Check sheet for the drawn part. Datum: minimum x, y, z corner. Units: mm. A direction names the side the tool comes from. Give positions to 0.01 mm unless a question says otherwise; leave off trailing zeros. Loops run counter-clockwise (first coordinate to the right, second up) from the corner with the lowest first, then second, coordinate; pieces in that order, holes last. Notation, with made-up numbers: (50.5, -24.75) - (86.5, -24.75) arc R21 ccw to (86.5, 2.25) - close; hole circle Ø11 at (41, -18). An arc over 180 degrees is marked (long way). One line per item, written item: value. Start each with the question number.
1. Sectioned sample at A-A (y = 3.5). Record the cut outline in (x, z), plus the area to 3 significant figures.
2. Sectioned sample at D-D (y = 0.5). Record the cut outline in (x, z).
3. Access from +Z, -Z, +X, -X, +Y, -Y to the whole of each face (thin tool, end or side, straight path). Record for the marked faces 1, 2 and 3.
4. Gauge pin test, flat ends, axial feed: pin 1 (1.6 mm diameter, centred on y = 4.5, z = 9, fed in from +X); pin 2 (2 mm diameter, centred on x = 7.5, y = 2.5, fed in from +Z). Record the tip position at first contact, or that the pin passes through.
5. Scan lines: L1, parallel to Z at x = 1, y = 3.5; L2, parallel to X at y = 2.5, z = 5.5; L3, parallel to Y at x = 0.5, z = 9. Record each from-to range of solid material in increasing order. Write a range as [from, to].
6. Mould release check, pull along X, two halves, no side actions. Record for the marked faces 4, 5, 6 and 7: pulls with the +X half, pulls with the -X half, needs draft (parallel to the pull), parting line crosses it, or undercut.
7. Sectioned sample at C-C (z = 10). Record the cut outline in (x, y), plus the area to 3 significant figures.
8. Sectioned sample at B-B (z = 12). Record the cut outline in (x, y).
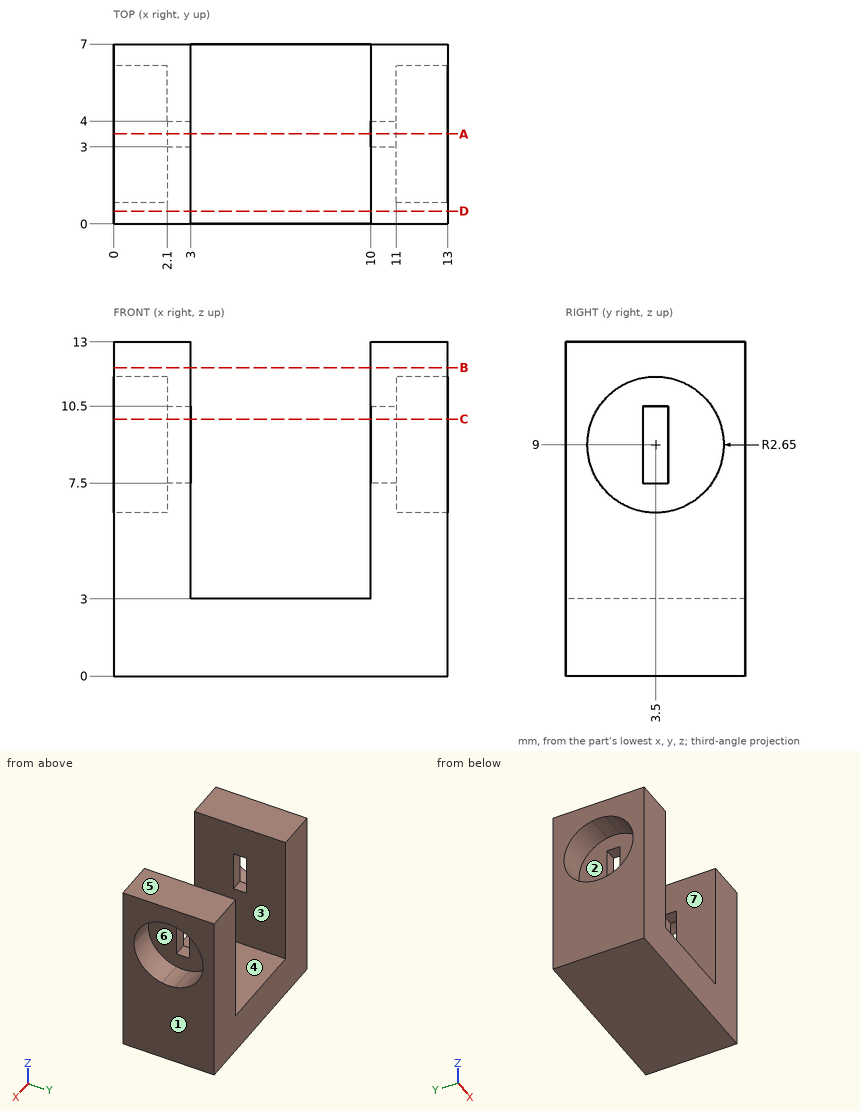
Results are:
1. outline: (0, 0) - (13, 0) - (13, 6.35) - (11, 6.35) - (11, 7.5) - (10, 7.5) - (10, 3) - (3, 3) - (3, 7.5) - (2.1, 7.5) - (2.1, 6.35) - (0, 6.35) - close; (0, 11.65) - (2.1, 11.65) - (2.1, 10.5) - (3, 10.5) - (3, 13) - (0, 13) - close; (10, 10.5) - (11, 10.5) - (11, 11.65) - (13, 11.65) - (13, 13) - (10, 13) - close
1. area: 71.6 mm^2
2. outline: (0, 0) - (13, 0) - (13, 13) - (10, 13) - (10, 3) - (3, 3) - (3, 13) - (0, 13) - close
3. face 1: +Z, -Z, +X, +Y, -Y
3. face 2: -X
3. face 3: +Z, +Y, -Y
4. pin 1: stops at x = 11
4. pin 2: stops at z = 3
5. L1: z = [0, 6.35], [11.65, 13]
5. L2: x = [0, 3], [10, 13]
5. L3: y = [0, 0.85], [6.15, 7]
6. face 4: undercut
6. face 5: needs draft
6. face 6: pulls with the +X half
6. face 7: undercut
7. outline: (0, 0) - (3, 0) - (3, 3) - (2.1, 3) - (2.1, 1.05) - (0, 1.05) - close; (0, 5.95) - (2.1, 5.95) - (2.1, 4) - (3, 4) - (3, 7) - (0, 7) - close; (10, 0) - (13, 0) - (13, 1.05) - (11, 1.05) - (11, 3) - (10, 3) - close; (10, 4) - (11, 4) - (11, 5.95) - (13, 5.95) - (13, 7) - (10, 7) - close
7. area: 20.0 mm^2
8. outline: (0, 0) - (3, 0) - (3, 7) - (0, 7) - close; (10, 0) - (13, 0) - (13, 7) - (10, 7) - close
